from build123d import *

# Parameters (mm, degrees)
SKETCH_1_W               = 10
SKETCH_1_H               = 10
SKETCH_1_W_2             = 8
SKETCH_1_H_2             = 8
EXTRUDE_1_DEPTH          = 200
CUT_EXTRUDE_1_DEPTH      = 201.31225624
CUT_EXTRUDE_1_DEPTH_BACK = 201.31225624
SKETCH_2_R               = 1.6
SKETCH_3_R               = 1.6
CUT_EXTRUDE_2_DEPTH      = 201.31225624
SKETCH_4_R               = 1.6
CUT_EXTRUDE_3_DEPTH      = 201.31225624


with BuildPart() as part:
    # ｽｹｯﾁ1 → ﾎﾞｽ - 押し出し1 (new body)
    with BuildSketch(Plane.XY):
        Rectangle(SKETCH_1_W, SKETCH_1_H)
        Rectangle(SKETCH_1_W_2, SKETCH_1_H_2, mode=Mode.SUBTRACT)
    extrude(amount=EXTRUDE_1_DEPTH)

    # ｽｹｯﾁ2 → ｶｯﾄ - 押し出し1 (cut, two sides: drawn at the far end of the back side and taken through both)
    with BuildSketch(Plane(origin=(5, 0, 0), x_dir=(0, 0, -1), z_dir=(1, 0, 0)).offset(-CUT_EXTRUDE_1_DEPTH_BACK)):
        with Locations(Location((-160, 0, 0), (0, 0, 90))):
            Circle(SKETCH_2_R)
        with Locations(Location((-40, 0, 0), (0, 0, 90))):
            Circle(SKETCH_2_R)
        with Locations(Location((-195, 0, 0), (0, 0, 90))):
            Circle(SKETCH_2_R)
        with Locations(Location((-5, 0, 0), (0, 0, 90))):
            Circle(SKETCH_2_R)
    extrude(amount=CUT_EXTRUDE_1_DEPTH + CUT_EXTRUDE_1_DEPTH_BACK, mode=Mode.SUBTRACT)

    # ｽｹｯﾁ3 → ｶｯﾄ - 押し出し2 (cut, through all)
    with BuildSketch(Plane(origin=(0, 5, 0), x_dir=(1, 0, 0), z_dir=(0, 1, 0))):
        with Locations(Location((0, -185, 0), (0, 0, 270))):
            Circle(SKETCH_3_R)
        with Locations(Location((0, -15, 0), (0, 0, 270))):
            Circle(SKETCH_3_R)
    extrude(amount=-CUT_EXTRUDE_2_DEPTH, mode=Mode.SUBTRACT)

    # ｽｹｯﾁ4 → ｶｯﾄ - 押し出し3 (cut, through all)
    with BuildSketch(Plane(origin=(0, 5, 0), x_dir=(1, 0, 0), z_dir=(0, 1, 0))):
        with Locations(Location((0, -50, 0), (0, 0, 270))):
            Circle(SKETCH_4_R)
        with Locations(Location((0, -150, 0), (0, 0, 270))):
            Circle(SKETCH_4_R)
    extrude(amount=-CUT_EXTRUDE_3_DEPTH, mode=Mode.SUBTRACT)


solid = part.part
The model under review builds one solid part; all positions refer to its coordinate system, in mm. A direction names the side the tool comes from. Round coordinates to 2 decimals unless told otherwise and drop trailing zeros. Loops run counter-clockwise (first coordinate to the right, second up) from the corner with the lowest first, then second, coordinate; pieces in that order, holes last. Notation, with made-up numbers: M 87,-5.5 L 131,-5.5 A16 ccw 131,-1.5 Z; hole C -23.5,-8 d3. An arc over 180 degrees is marked long. Answer as CSV lines item,"result". Start each with the question number.
Item 1: Insertion check: P1, Ø1.9, axis at x = 0, z = 15, coming from the -Y side. The pin has a flat end and moves straight along its axis. Give the tip position at first contact, or say it passes through.
Item 2: For faces 1 (the face through (4, 0, 99)), 2 (the face through (-0.61, -4.49, 151.48)), list the 3-axis set-ups (+Z, -Z, +X, -X, +Y, -Y) from which the entire face can be reached by the end or side of a thin tool; tool diameter is ignored.
Item 3: Mouldability with a two-part tool opening along Z and no side actions: class faces 3 (the face through (-4.5, 0.1, 200)), 4 (the face through (-4.51, 0.74, 38.58)), 5 (the face through (0, 5, 99)) as released by +Z, released by -Z, zero draft, split by the parting line, or undercut.
Item 4: Consider section B-B (y = 0). State how many separate pieces and enclosed holes the cut face has, then the cut area to 3 significant figures.
Item 5: Wall thickness on line 1 (Z direction, x = 4.5, y = 0); line 2 (Y direction, x = -1.5, z = 137): over which ranges is each line inside the solid? List them lowest first. Write a range as [from, to].
Item 6: Consider section A-A (z = 107.5). Write out the cut boundary in (x, y), then the cut area to 3 significant figures.
Answer:
1,P1,"passes through"
2,face 1,"+Z, -Z"
2,face 2,"+Y, -Y"
3,face 3,"released by +Z"
3,face 4,"undercut"
3,face 5,"zero draft"
4,separate pieces,"10"
4,enclosed holes,"0"
4,area,"374 mm^2"
5,line 1,"z = [0, 3.4], [6.6, 38.4], [41.6, 158.4], [161.6, 193.4], [196.6, 200]"
5,line 2,"y = [-5, -4], [4, 5]"
6,outline,"M -5,-5 L 5,-5 L 5,5 L -5,5 Z; hole M -4,-4 L 4,-4 L 4,4 L -4,4 Z"
6,area,"36.0 mm^2"
